```python
from build123d import *

# Parameters (mm, degrees)
EXTRUDE_DEPTH = 5
FILLET_R      = 1


with BuildPart() as part:
    # Sketch → Extrude (new body)
    with BuildSketch(Plane.XY):
        with BuildLine():
            Line((0, 0), (200, 0))
            Line((200, 5), (200, 0))
            Line((23.923846, 5), (200, 5))
            ThreePointArc((23.264837, 7.176558), (22.786778, 5.843768), (23.923846, 5))
            Line((35, 15), (23.264837, 7.176558))
            Line((25, 15), (35, 15))
            Line((0, 0), (25, 15))
        make_face()
    extrude(amount=EXTRUDE_DEPTH)

    # Fillet
    fillet_edges = [part.edges().sort_by_distance(p)[0] for p in [
        (0, 0, 2.5),
        (200, 0, 2.5),
        (100, 0, 0),
        (100, 0, 5),
        (200, 5, 2.5),
        (200, 2.5, 0),
        (200, 2.5, 5),
        (111.961923, 5, 0),
        (111.961923, 5, 5),
        (22.786778, 5.843768, 0),
        (22.786778, 5.843768, 5),
        (29.132419, 11.088279, 0),
        (29.132419, 11.088279, 5),
        (25, 15, 2.5),
        (30, 15, 0),
        (30, 15, 5),
        (12.5, 7.5, 0),
        (12.5, 7.5, 5),
    ]]
    fillet(fillet_edges, radius=FILLET_R)


solid = part.part
```
Can you work these out from the model? Positions are in its coordinate system, mm. A direction names the side the tool comes from. Coordinates: 2 decimals unless noted, no trailing zeros. Loops run counter-clockwise (first coordinate to the right, second up) from the corner with the lowest first, then second, coordinate; pieces in that order, holes last.
1) Which directions (+Z, -Z, +X, -X, +Y, -Y) give clear straight access to the entire face, cutting with the end or side of a thin tool? Please do faces 1 (the cylindrical face through (28.89, 11.27, 0.3)), 2 (the cylindrical face through (14.228, 8.204, 4.699)), 3 (the flat face through (29, 11, 2)), 4 (the flat face through (13.78, 8.27, 2.48)), 5 (the cylindrical face through (28.89, 11.27, 4.7)).
2) For pin 1 (3 mm diameter, centred on y = 3.5, z = 4, fed in from -X), with a flat end and sliding along its axis, tell me the tip position at first contact or that it passes through.
3) Imagine slicing it at A-A on x = 177.5. List the corners of the cut face in (y, z) for me, plus the area to 3 significant figures.
4) Imagine slicing it at B-B on z = 1.8. List the corners of the cut face in (x, y) for me.
5) I need wall thicknesses on probe 1 along Y at (x, z) = (179.5, 2.45); probe 2 along Y at (x, z) = (34, 4.3); probe 3 along X at (y, z) = (8.5, 4). Which ranges of each line are inside material? Lowest first, please.
Completed:
1. face 1: -Z, +X
1. face 2: +Z, -X, +Y
1. face 3: +Z, -Z, +X
1. face 4: +Z, -Z, -X, +Y
1. face 5: +Z, +X
2. pin 1: stops at x = 3.33
3. outline: (0, 1) arc R1 ccw to (1, 0) - (4, 0) arc R1 ccw to (5, 1) - (5, 4) arc R1 ccw to (4, 5) - (1, 5) arc R1 ccw to (0, 4) - close
3. area: 24.1 mm2
4. outline: (3.1, 1.86) arc R1 ccw to (3.61, 0) - (199, 0) arc R1 ccw to (200, 1) - (200, 4) arc R1 ccw to (199, 5) - (23.92, 5) arc R1.19 cw to (23.26, 7.18) - (35, 15) - (25.28, 15) arc R1 ccw to (24.76, 14.86) - close
5. probe 1: y = 0 to 5
5. probe 2: y = 0.05 to 4.95, 14.39 to 14.95
5. probe 3: x = 14.17 to 25.25
